Part model, mm, in its own coordinate system. A direction names the side the tool comes from. Give positions to 0.01 mm unless a question says otherwise; leave off trailing zeros. Write each loop counter-clockwise with the first axis right and the second up, starting at its lowest first coordinate (ties: lowest second). Pieces come first, ordered by that corner, then holes.
```python
from build123d import *

# Parameters (mm, degrees)
SKETCH1_W           = 9.6
SKETCH1_H           = 16.8
SKETCH1_R           = 1.5
BOSS_EXTRUDE1_DEPTH = 3.2
SKETCH3_W           = 16.8
SKETCH3_H           = 3.2
BOSS_EXTRUDE2_DEPTH = 3.2
SKETCH4_W           = 6.522228594
SKETCH4_H           = 1.6
BOSS_EXTRUDE3_DEPTH = 4.8
SKETCH5_W           = 6.289556992
SKETCH5_H           = 1.6
BOSS_EXTRUDE4_DEPTH = 4.8


with BuildPart() as part:
    # Sketch1 → Boss-Extrude1 (new body)
    with BuildSketch(Plane(origin=(0, 0, 0), x_dir=(1, 0, 0), z_dir=(0, 1, 0))):
        with Locations((4.8, -8.4)):
            Rectangle(SKETCH1_W, SKETCH1_H)
        with Locations(Location((4.8, -12, 0), (0, 0, 270))):
            Circle(SKETCH1_R, mode=Mode.SUBTRACT)
    extrude(amount=BOSS_EXTRUDE1_DEPTH)

    # Sketch3 → Boss-Extrude2 (add)
    with BuildSketch(Plane.ZY):
        with Locations((8.4, 1.6)):
            Rectangle(SKETCH3_W, SKETCH3_H)
    extrude(amount=BOSS_EXTRUDE2_DEPTH)

    # Sketch4 → Boss-Extrude3 (add)
    with BuildSketch(Plane(origin=(0, 0, 0), x_dir=(-1, 0, 0), z_dir=(0, -1, 0))):
        with Locations((-0.061114297, -15.2)):
            Rectangle(SKETCH4_W, SKETCH4_H)
    extrude(amount=BOSS_EXTRUDE3_DEPTH)

    # Sketch5 → Boss-Extrude4 (add)
    with BuildSketch(Plane(origin=(0, 0, 0), x_dir=(-1, 0, 0), z_dir=(0, -1, 0))):
        with Locations((0.055221504, -0.8)):
            Rectangle(SKETCH5_W, SKETCH5_H)
    extrude(amount=BOSS_EXTRUDE4_DEPTH)


solid = part.part
```
1) Wall check: L1, parallel to Z at x = -0.5, y = -0.5; L2, parallel to X at y = 1.25, z = 12; L3, parallel to Z at x = 4.75, y = 2.5. Give the ranges that are in metal, low to high.
Answers follow:
L1: z = 0 to 1.6, 14.4 to 16
L2: x = -3.2 to 3.3, 6.3 to 9.6
L3: z = 0 to 10.5, 13.5 to 16.8
2) Saw through at C-C, the plane x = 0.75. Write the cut outline in (y, z).
Answers follow:
outline: (-4.8, 0) - (3.2, 0) - (3.2, 16.8) - (0, 16.8) - (0, 16) - (-4.8, 16) - (-4.8, 14.4) - (0, 14.4) - (0, 1.6) - (-4.8, 1.6) - close
3) Saw through at D-D, the plane y = 0.25. Write the cut outline in (x, z), then the cut area to 3 significant figures.
Answers follow:
outline: (-3.2, 0) - (9.6, 0) - (9.6, 16.8) - (-3.2, 16.8) - close; hole circle Ø3 at (4.8, 12)
area: 208 mm2
4) Two-plate mould, pull along X, no slides. Class faces 6 (the face through (9.6, 2, 9)), 7 (the face through (-3.2, 1, 9)), 8 (the face through (0, -2, 14.4)), 9 (the face through (6.287, 1.578, 11.805)): +X half, -X half, draft (parallel to the pull), parting line (faces both ways), or undercut.
Answers follow:
face 6: +X half
face 7: -X half
face 8: draft
face 9: undercut
5) Saw through at B-B, the plane x = 6. Write the cut outline in (y, z).
Answers follow:
outline: (0, 0) - (3.2, 0) - (3.2, 11.1) - (0, 11.1) - close; (0, 12.9) - (3.2, 12.9) - (3.2, 16.8) - (0, 16.8) - close
6) Saw through at A-A, the plane z = 12. Write the cut outline in (x, y).
Answers follow:
outline: (-3.2, 0) - (3.3, 0) - (3.3, 3.2) - (-3.2, 3.2) - close; (6.3, 0) - (9.6, 0) - (9.6, 3.2) - (6.3, 3.2) - close
7) Pin check, flat tips, straight feed: pin 1 Ø1.4 at (x, y) = (-0.5, -2) entering from +Z; pin 2 Ø3 at (x, y) = (1, 2) entering from -Z; pin 3 Ø1.3 at (y, z) = (-3, 15) entering from +X; pin 4 Ø2 at (x, z) = (7.5, 8.5) entering from -Y. Stop position of each tip, or through.
Answers follow:
pin 1: stops at z = 16
pin 2: stops at z = 0
pin 3: stops at x = 3.32
pin 4: stops at y = 0
8) 3-axis set-ups, long thin cutter, end or side, ignore diameter. For faces 1 (the face through (0, -4.8, 15)), 2 (the face through (0, -2, 1.6)), 3 (the face through (0, -2, 16)), 4 (the face through (3.322, -2, 15)), 5 (the face through (3.09, -2, 1)): which of +Z, -Z, +X, -X, +Y, -Y reach the whole face in a straight line?
Answers follow:
face 1: +Z, -Z, +X, -X, -Y
face 2: +X, -X, -Y
face 3: +Z, +X, -X, -Y
face 4: +Z, -Z, +X, -Y
face 5: -Z, +X, -Y
